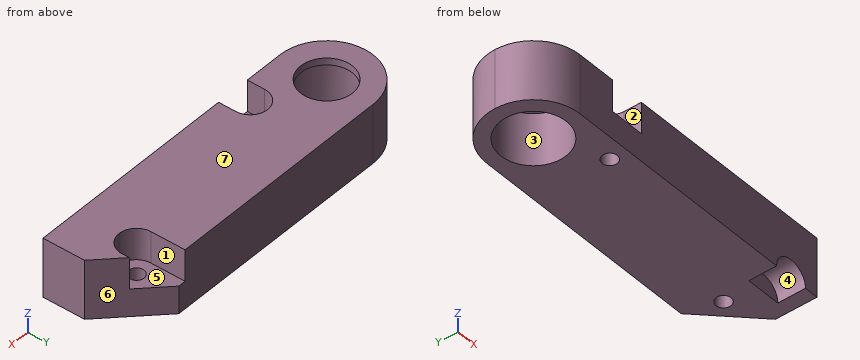
from build123d import *

# Parameters (mm, degrees)
F0_R     = 1.7272
F0_R_2   = 5.9124977
F1_DEPTH = 1.5875
F2_R     = 1.7272
F2_R_2   = 7.5
F3_DEPTH = 12
F5_DEPTH = 6.35
F6_R     = 10.674988
F7_W     = 7.9375
F7_H     = 7.9375
F8_DEPTH = 7.2375014
F9_R     = 3.96874


# Not quite as in the source:
# - a fillet or chamfer is up to 0.001 mm smaller than in the source, because OpenCascade refuses the exact size


with BuildPart() as f1:
    # F0 (on Top) → F1 (new body)
    with BuildSketch(Plane.XY):
        Polygon((64.3750046, 0), (0, 0), (0, -21.3499954), (76.2, -21.3499954), (76.2, -11.8249954), align=None)
        with Locations((23.692892633, -17.3812454)):
            Circle(F0_R, mode=Mode.SUBTRACT)
        with Locations((10.6749977, -10.6749977)):
            Circle(F0_R_2, mode=Mode.SUBTRACT)
        with Locations((66.6185899243, -7.8562454)):
            Circle(F0_R, mode=Mode.SUBTRACT)
    extrude(amount=F1_DEPTH)

    # F2 (on face) → F3 (join)
    with BuildSketch(Plane(origin=(0, 0, 0), x_dir=(1, 0, 0), z_dir=(0, 0, -1))):
        Polygon((0, 0), (64.3750046, 0), (76.2, 11.8249954), (76.2, 21.3499954), (0, 21.3499954), align=None)
        with Locations((66.6185899243, 7.8562454)):
            Circle(F2_R, mode=Mode.SUBTRACT)
        with Locations((10.6749977, 10.6749977)):
            Circle(F2_R_2, mode=Mode.SUBTRACT)
        with Locations((23.692892633, 17.3812454)):
            Circle(F2_R, mode=Mode.SUBTRACT)
    extrude(amount=F3_DEPTH)

    # F4 (on face) → F5 (cut)
    with BuildSketch(Plane.XZ.offset(21.3499954)):
        with BuildLine():
            Line((65.025, -12), (73.025, -12))
            ThreePointArc((73.025, -12), (69.025, -8), (65.025, -12))
        make_face()
    extrude(amount=-F5_DEPTH, mode=Mode.SUBTRACT)

    # F6 (radius 10.6749977 in the source; OpenCascade refuses exactly that, so slightly less here)
    f6_edges = [f1.edges().sort_by_distance(p)[0] for p in [
        (0, -21.349995, -5.20625),
        (0, 0, -5.20625),
    ]]
    fillet(f6_edges, radius=F6_R)

    # F7 (on face) → F8 (cut)
    with BuildSketch(Plane.XY.offset(1.5875)):
        with Locations((23.692892633, -17.3812454)):
            Rectangle(F7_W, F7_H)
        Polygon((64.3750046, 0), (62.6498399243, 0), (62.6498399243, -11.8249954), (70.5873399243, -11.8249954), (70.5873399243, -6.2123353243), align=None)
    extrude(amount=-F8_DEPTH, mode=Mode.SUBTRACT)

    # F9 (radius 3.96875 in the source; OpenCascade refuses exactly that, so slightly less here)
    f9_edges = [f1.edges().sort_by_distance(p)[0] for p in [
        (27.661643, -13.412495, -2.031251),
        (19.724143, -13.412495, -2.031251),
        (62.64984, -11.824995, -2.031251),
        (70.58734, -11.824995, -2.031251),
    ]]
    fillet(f9_edges, radius=F9_R)


solid = f1.part
The listing builds one solid part. Answer for the finished solid, in the listing's coordinates (mm). Face numbers are marked on the shaded views. A direction names the side the tool comes from. Coordinates: 2 decimals unless noted, no trailing zeros. Answer in a Markdown table with one row per item. Add a question column.
Item 1: Find the intervals of material crossed by L1, parallel to X at y = -14, z = -1.75; L2, parallel to X at y = -9, z = -2.25 (3 decimals); L3, parallel to Z at x = 13, y = -17.25, in increasing order. Write a range as from..to.
Item 2: Determine the mould class of the marked faces 5, 6 and 7 for opening direction X: +X half, -X half, draft (parallel to the pull), parting line (faces both ways), or undercut.
Item 3: Which of the six approach directions +Z, -Z, +X, -X, +Y, -Y give full straight-line access (tool end or side, diameter ignored) to the marked faces 1, 2, 3 and 4?
Item 4: Each of these flat-tipped pins is pushed along its axis until it touches: P1, Ø8, axis at y = -5.5, z = -3.5, coming from the +X side (3 decimals); P2, Ø3, axis at x = 69, z = -10, coming from the -Y side; P3, Ø2.5, axis at x = 67, y = -7, coming from the +Z side; P4, Ø2, axis at x = 23.69, y = -17.38, coming from the -Z side. Where does it stop, or does it pass through?
Result set:
| question | item | result |
|---|---|---|
| 1 | L1 | x = 0.53..3.95, 17.4..21.61, 25.77..76.2 |
| 1 | L2 | x = 0.132..3.364, 17.986..62.818, 70.419..73.375 |
| 1 | L3 | z = 0..1.59 |
| 2 | face 5 | undercut |
| 2 | face 6 | +X half |
| 2 | face 7 | draft |
| 3 | face 1 | +Z, +Y |
| 3 | face 2 | +Z, -Y |
| 3 | face 3 | -Z |
| 3 | face 4 | -Z, -Y |
| 4 | P1 | stops at x = 73.875 |
| 4 | P2 | stops at y = -15 |
| 4 | P3 | stops at z = -5.65 |
| 4 | P4 | passes through |
